```python
from build123d import *

# Parameters (mm, degrees)
SKETCH_1_R          = 9
EXTRUDE_1_DEPTH     = 2
SKETCH_2_R          = 3.5
SKETCH_2_R_2        = 2
EXTRUDE_2_DEPTH     = 2
SKETCH_3_R          = 1.1
CUT_EXTRUDE_1_DEPTH = 14.341664064


with BuildPart() as part:
    # 草图1 → 凸台-拉伸1 (new body)
    with BuildSketch(Plane(origin=(0, 0, 0), x_dir=(1, 0, 0), z_dir=(0, 1, 0))):
        with Locations(Location((0, 0, 0), (0, 0, 270))):
            Circle(SKETCH_1_R)
    extrude(amount=EXTRUDE_1_DEPTH)

    # 草图2 → 凸台-拉伸2 (add)
    with BuildSketch(Plane(origin=(0, 2, 0), x_dir=(1, 0, 0), z_dir=(0, 1, 0))):
        with Locations(Location((0, 0, 0), (0, 0, 270))):
            Circle(SKETCH_2_R)
        with Locations(Location((0, 0, 0), (0, 0, 270))):
            Circle(SKETCH_2_R_2, mode=Mode.SUBTRACT)
    extrude(amount=EXTRUDE_2_DEPTH)

    # 草图3 → 切除-拉伸1 (cut, through all)
    with BuildSketch(Plane.XZ):
        with Locations(Location((0, 6.5, 0), (0, 0, 270))):
            Circle(SKETCH_3_R)
        with Locations(Location((4.596194078, 4.596194078, 0), (0, 0, 270))):
            Circle(SKETCH_3_R)
        with Locations(Location((6.5, 0, 0), (0, 0, 270))):
            Circle(SKETCH_3_R)
        with Locations(Location((4.596194078, -4.596194078, 0), (0, 0, 270))):
            Circle(SKETCH_3_R)
        with Locations(Location((0, -6.5, 0), (0, 0, 270))):
            Circle(SKETCH_3_R)
        with Locations(Location((-4.596194078, -4.596194078, 0), (0, 0, 270))):
            Circle(SKETCH_3_R)
        with Locations(Location((-6.5, 0, 0), (0, 0, 270))):
            Circle(SKETCH_3_R)
        with Locations(Location((-4.596194078, 4.596194078, 0), (0, 0, 270))):
            Circle(SKETCH_3_R)
    extrude(amount=-CUT_EXTRUDE_1_DEPTH, mode=Mode.SUBTRACT)


solid = part.part
```
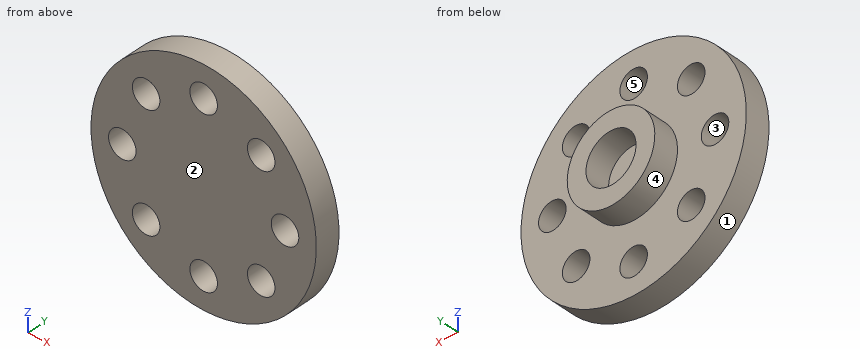
Read the model definition and answer for the solid it produces. Units are mm, in the model's axes. Face numbers are marked on the shaded views. A direction names the side the tool comes from. Coordinates: 2 decimals unless noted, no trailing zeros. Write each loop counter-clockwise with the first axis right and the second up, starting at its lowest first coordinate (ties: lowest second). Pieces come first, ordered by that corner, then holes. Notation, with made-up numbers: (86, 59.5) -> (128, 59.5) arc R14 ccw to (128, 69.5) -> close; hole circle Ø9 at (16.5, 73.25). An arc over 180 degrees is marked (long way). Return JSON: item names as keys, results as strings.
1. Each of these flat-tipped pins is pushed along its axis until it touches: P1, Ø1.2, axis at x = 0, z = 0.5, coming from the +Y side; P2, Ø2, axis at y = 3.5, z = 4, coming from the +X side. Where does it stop, or does it pass through?
Found:
{"P1": "y = 2", "P2": "x = 1.8"}
2. Determine the mould class of the marked faces 1, 2 and 3 for opening direction Z: pulls with the +Z half, pulls with the -Z half, needs draft (parallel to the pull), parting line crosses it, or undercut.
Found:
{"face 1": "parting line crosses it", "face 2": "needs draft", "face 3": "undercut"}
3. A cutting plane is placed at D-D (y = 1.4). Give the number of separate pieces and of enclosed holes in the cut face, and give its area (3 significant figures).
Found:
{"separate pieces": "1", "enclosed holes": "8", "area": "224 mm2"}
4. A cutting plane is placed at A-A (z = 0). Determine the outline of the cut face in (x, y).
Found:
{"outline": "(-9, 0) -> (-7.6, 0) -> (-7.6, 2) -> (-9, 2) -> close; (-5.4, 0) -> (5.4, 0) -> (5.4, 2) -> (3.5, 2) -> (3.5, 4) -> (2, 4) -> (2, 2) -> (-2, 2) -> (-2, 4) -> (-3.5, 4) -> (-3.5, 2) -> (-5.4, 2) -> close; (7.6, 0) -> (9, 0) -> (9, 2) -> (7.6, 2) -> close"}
5. A tool of negligible diameter and unlimited length cuts with its end or side. For the marked faces 4 and 5, from which of +Z, -Z, +X, -X, +Y, -Y can it reach the whole face along a straight path? Write none if from no direction.
Found:
{"face 4": "+Y", "face 5": "+Y, -Y"}
6. A cutting plane is placed at B-B (x = 0). Determine the outline of the cut face in (y, z).
Found:
{"outline": "(0, -9) -> (2, -9) -> (2, -7.6) -> (0, -7.6) -> close; (0, -5.4) -> (2, -5.4) -> (2, -3.5) -> (4, -3.5) -> (4, -2) -> (2, -2) -> (2, 2) -> (4, 2) -> (4, 3.5) -> (2, 3.5) -> (2, 5.4) -> (0, 5.4) -> close; (0, 7.6) -> (2, 7.6) -> (2, 9) -> (0, 9) -> close"}
7. Find the intervals of material crossed by line 1 along X through (y, z) = (0.4, 0); line 2 along X through (y, z) = (1.5, -5.5); line 3 along X through (y, z) = (2.75, 0), in increasing order. Write a range as from..to.
Found:
{"line 1": "-9..-7.6, -5.4..5.4, 7.6..9", "line 2": "-7.12..-5.22, -3.97..-0.46, 0.46..3.97, 5.22..7.12", "line 3": "-3.5..-2, 2..3.5"}
8. A cutting plane is placed at C-C (z = -6.5). Determine the outline of the cut face in (x, y), and give its area (3 significant figures).
Found:
{"outline": "(-6.22, 0) -> (-1.1, 0) -> (-1.1, 2) -> (-6.22, 2) -> close; (1.1, 0) -> (6.22, 0) -> (6.22, 2) -> (1.1, 2) -> close", "area": "20.5 mm2"}
